Here's how the part is built. I have some questions about the finished solid (model axes, mm). A direction names the side the tool comes from. Give positions to 0.01 mm unless a question says otherwise; leave off trailing zeros. Write each loop counter-clockwise with the first axis right and the second up, starting at its lowest first coordinate (ties: lowest second). Pieces come first, ordered by that corner, then holes. Notation, with made-up numbers: (-5.5, -31) -> (40.5, -31) arc R21 ccw to (40.5, -13) -> close; hole circle Ø4 at (37, 75). An arc over 180 degrees is marked (long way). Return JSON: item names as keys, results as strings.
Autodesk Fusion 360 part; units mm, degrees
sketch "Skizze1" plane through (0, 0, 0) normal (0, 0, 1) x (1, 0, 0)
  line L0 (0, 0) -> (60, 0)
  line L1 (60, 0) -> (60, 34)
  line L2 (60, 34) -> (0, 34)
  line L3 (0, 34) -> (0, 0)
  circle A0 centre (4, 4.5) radius 1.5
  circle A1 centre (55.5, 4.5) radius 1.5
  circle A2 centre (55.5, 4.5) radius 1.5
  circle A3 centre (4, 4.5) radius 1.5
  line L4 (0, 0) -> (60, 0)
  circle A4 centre (55.5, 29.5) radius 1.5
  circle A5 centre (4, 29.5) radius 1.5
  circle A6 centre (55.5, 29.5) radius 1.5
  circle A7 centre (4, 29.5) radius 1.5
  circle A8 centre (13, 28.5) radius 1
  circle A9 centre (13, 5.5) radius 1
  circle A10 centre (36.5, 5.5) radius 1
  circle A11 centre (36.5, 28.5) radius 1
  line L5 (11, 23) -> (15, 23)
  line L6 (15, 23) -> (15, 11)
  line L7 (15, 11) -> (11, 11)
  line L8 (11, 11) -> (11, 23)
  circle A12 centre (49, 17.25) radius 3.5
  point P0 (51.5, 0)
  point P1 (51.5, 0)
  point P2 (51.5, 0)
  point P3 (51.5, 0)
  dimension "d1" = 60
  dimension "d2" = 34
  dimension "d3" = 3
  dimension "d4" = 3
  dimension "d5" = 60
  dimension "d6" = 3
  dimension "d7" = 3
  dimension "d8" = 3
  dimension "d9" = 3
  dimension "d10" = 3
  dimension "d11" = 3
  dimension "d12" = 2
  dimension "d13" = 2
  dimension "d14" = 2
  dimension "d15" = 2
  dimension "d16" = 7
extrude "Extrusion1" add sketch "Skizze1" along normal blind 2.5
1. For pin 1 Ø1.8 at (x, y) = (13, 5.5) entering from -Z, with a flat end and sliding along its axis, tell me the tip position at first contact or that it passes through.
Taken from the geometry:
{"pin 1": "passes through"}
2. If I drill on line 1 (Y direction, x = 13, z = 1.8); line 2 (X direction, y = 15, z = 0.75); line 3 (X direction, y = 18.5, z = 0.3), over which ranges is the centre line in solid material (lowest first)? Write a range as [from, to].
Taken from the geometry:
{"line 1": "y = [0, 4.5], [6.5, 11], [23, 27.5], [29.5, 34]", "line 2": "x = [0, 11], [15, 46.32], [51.68, 60]", "line 3": "x = [0, 11], [15, 45.73], [52.27, 60]"}
3. If we mould it in two halves opening along X, with no side actions, what happens to faces 1 (the face through (60, 17, 1)), 2 (the face through (15, 17, 1)), 3 (the face through (30, 34, 1)), 4 (the face through (0, 17, 1))? For each: released by +X, released by -X, zero draft, split by the parting line, or undercut.
Taken from the geometry:
{"face 1": "released by +X", "face 2": "undercut", "face 3": "zero draft", "face 4": "released by -X"}
4. Suppose I cut it at D-D, the plane x = 49. List the corners of the cut face in (y, z) for me, and give its area (3 significant figures).
Taken from the geometry:
{"outline": "(0, 0) -> (13.75, 0) -> (13.75, 2.5) -> (0, 2.5) -> close; (20.75, 0) -> (34, 0) -> (34, 2.5) -> (20.75, 2.5) -> close", "area": "67.5 mm²"}
5. Suppose I cut it at C-C, the plane z = 1.5. Count the separate pieces of the cut face and the enclosed holes in it, and give its area (3 significant figures).
Taken from the geometry:
{"separate pieces": "1", "enclosed holes": "10", "area": "1,910 mm²"}
6. Suppose I cut it at B-B, the plane x = 55.5. List the corners of the cut face in (y, z) for me.
Taken from the geometry:
{"outline": "(0, 0) -> (3, 0) -> (3, 2.5) -> (0, 2.5) -> close; (6, 0) -> (28, 0) -> (28, 2.5) -> (6, 2.5) -> close; (31, 0) -> (34, 0) -> (34, 2.5) -> (31, 2.5) -> close"}
7. Suppose I cut it at A-A, the plane x = 13. List the corners of the cut face in (y, z) for me.
Taken from the geometry:
{"outline": "(0, 0) -> (4.5, 0) -> (4.5, 2.5) -> (0, 2.5) -> close; (6.5, 0) -> (11, 0) -> (11, 2.5) -> (6.5, 2.5) -> close; (23, 0) -> (27.5, 0) -> (27.5, 2.5) -> (23, 2.5) -> close; (29.5, 0) -> (34, 0) -> (34, 2.5) -> (29.5, 2.5) -> close"}
8. Which directions (+Z, -Z, +X, -X, +Y, -Y) give clear straight access to the entire face, cutting with the end or side of a thin tool? Please do faces 5 (the face through (30, 17, 0)), 6 (the face through (13, 23, 1)).
Taken from the geometry:
{"face 5": "-Z, +X, -X, +Y, -Y", "face 6": "+Z, -Z"}
